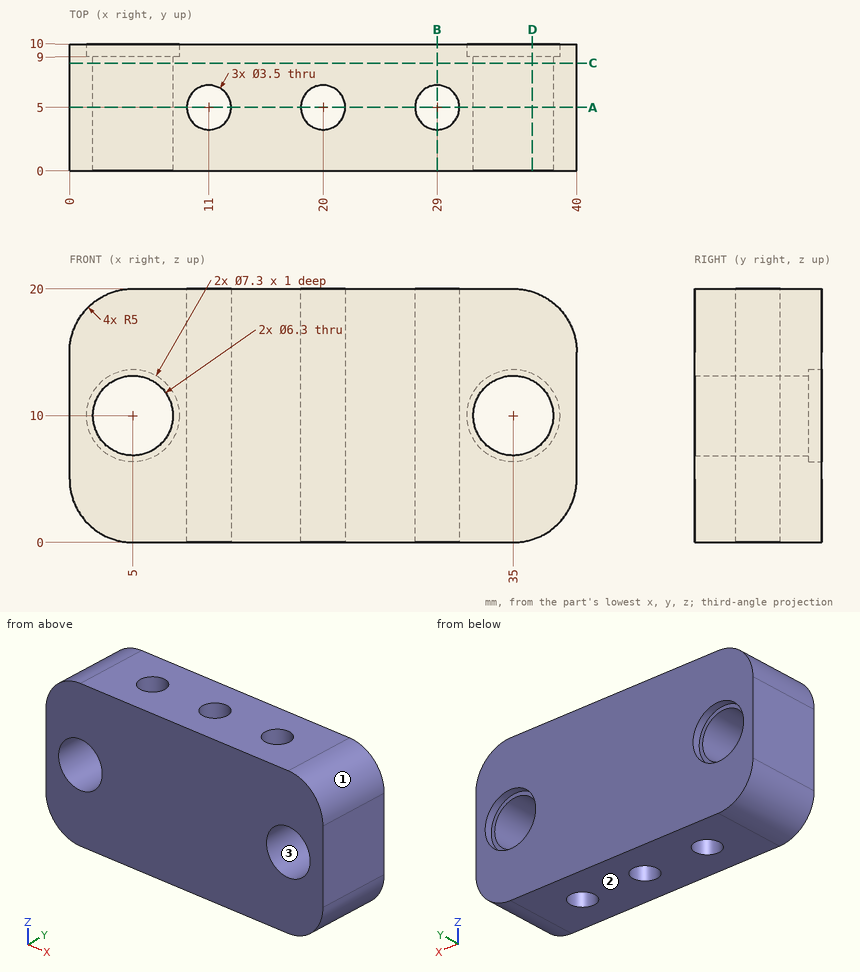
Job drawing, mm, ordinate dimensions from the low corner. One solid piece. Coordinates: 2 decimals unless noted, no trailing zeros. Order: outer loops, then holes, each group sorted by start corner. A loop starts at its lowest first (then second) coordinate and runs counter-clockwise, first axis right, second up. Notation, with made-up numbers: (-0.75, 88.5) -> (15.25, 88.5) arc R23 ccw to (15.25, 120.5) -> close; hole circle Ø11 at (-35.75, 32.5). An arc over 180 degrees is marked (long way). Answer in a Markdown table with one row per item. Add a question column.
Q1. Band-saw the part on B-B, the plane x = 29. List the corners of the cut face in (y, z), then the cut area to 3 significant figures.
Q2. Band-saw the part on A-A, the plane y = 5. List the corners of the cut face in (x, z).
Q3. Drop a flat-ended pin along its axis: pin 1 (2 mm diameter, centred on x = 29, y = 5, fed in from +Z). Give the stop position or say it passes through.
Q4. Band-saw the part on C-C, the plane y = 8.5. List the corners of the cut face in (x, z).
Q5. Wall check: line 1 along X through (y, z) = (9.7, 10); line 2 along Y through (x, z) = (20, 10); line 3 along X through (y, z) = (4.5, 2). Give the ranges that are in metal, low to high. Write a range as [from, to].
Q6. Mould opens along Z. For the marked faces 1, 2 and 3 say: +Z half, -Z half, draft (parallel to the pull), parting line (faces both ways), or undercut.
Q7. Band-saw the part on D-D, the plane x = 36.5. List the corners of the cut face in (y, z), then the cut area to 3 significant figures.
Answers follow:
| question | item | result |
|---|---|---|
| 1 | outline | (0, 0) -> (3.25, 0) -> (3.25, 20) -> (0, 20) -> close; (6.75, 0) -> (10, 0) -> (10, 20) -> (6.75, 20) -> close |
| 1 | area | 130 mm^2 |
| 2 | outline | (0, 5) arc R5 ccw to (5, 0) -> (9.25, 0) -> (9.25, 20) -> (5, 20) arc R5 ccw to (0, 15) -> close; (12.75, 0) -> (18.25, 0) -> (18.25, 20) -> (12.75, 20) -> close; (21.75, 0) -> (27.25, 0) -> (27.25, 20) -> (21.75, 20) -> close; (30.75, 0) -> (35, 0) arc R5 ccw to (40, 5) -> (40, 15) arc R5 ccw to (35, 20) -> (30.75, 20) -> close; hole circle Ø6.3 at (5, 10); hole circle Ø6.3 at (35, 10) |
| 3 | pin 1 | through |
| 4 | outline | (0, 5) arc R5 ccw to (5, 0) -> (35, 0) arc R5 ccw to (40, 5) -> (40, 15) arc R5 ccw to (35, 20) -> (5, 20) arc R5 ccw to (0, 15) -> close; hole circle Ø6.3 at (5, 10); hole circle Ø6.3 at (35, 10) |
| 5 | line 1 | [0, 1.35], [8.65, 31.35], [38.65, 40] |
| 5 | line 2 | [0, 3.25], [6.75, 10] |
| 5 | line 3 | [1, 9.32], [12.68, 18.32], [21.68, 27.32], [30.68, 39] |
| 6 | face 1 | +Z half |
| 6 | face 2 | -Z half |
| 6 | face 3 | undercut |
| 7 | outline | (0, 0.23) -> (10, 0.23) -> (10, 6.67) -> (9, 6.67) -> (9, 7.23) -> (0, 7.23) -> close; (0, 12.77) -> (9, 12.77) -> (9, 13.33) -> (10, 13.33) -> (10, 19.77) -> (0, 19.77) -> close |
| 7 | area | 139 mm^2 |
